The listing builds one solid part. Answer for the finished solid, in the listing's coordinates (mm). A direction names the side the tool comes from. Give positions to 0.01 mm unless a question says otherwise; leave off trailing zeros. Order: outer loops, then holes, each group sorted by start corner. A loop starts at its lowest first (then second) coordinate and runs counter-clockwise, first axis right, second up. Notation, with made-up numbers: (47, 27) - (53, 27) arc R12 cw to (53, 37) - close; hole circle Ø3 at (-23.5, -4.5). An arc over 180 degrees is marked (long way). Use a Markdown table: item, result. Add a question column.
1) Find section A-A, the plane z = 1.25. Determine the outline of the cut face in (x, y), plus the area to 3 significant figures.
2) The mould has two halves that part along Y. Classify faces 1 (the face through (187.854, -58.176, 1.521)), 2 (the face through (50, 98, 3)), 3 (the face through (60, 93, 3)): released by +Y, released by -Y, zero draft, split by the parting line, or undercut.
3) Find section B-B, the plane x = 170.5. Determine the outline of the cut face in (y, z), plus the area to 3 significant figures.
4) Flat-ended cylindrical pins translate along their axes: pin 1 (6 mm diameter, centred on x = 93.5, y = -63.5, fed in from +Z); pin 2 (6 mm diameter, centred on x = 153.5, y = 17, fed in from +Z); pin 3 (3 mm diameter, centred on x = 39.5, y = 57.5, fed in from +Z); pin 4 (0.9 mm diameter, centred on x = 12.5, y = 111, fed in from -Z). Find the tip coordinate at first contact, or state that the pin passes through.
5) Straight lines are drawn through the part: line 1 (Y direction, x = 15.5, z = 6.75); line 2 (Y direction, x = 190, z = 2.2); line 3 (X direction, y = -15.5, z = 4.75). For each, find the intervals that lie inside material, in ascending order.
6) For faces 4 (the face through (122.854, -58.176, 1.521)), 5 (the face through (161, -50, 3)), 6 (the face through (44, 110, 6)), 7 (the face through (47.15, 109.99, 3.71)), 8 (the face through (43.275, 109.449, 5.507)), determine the directions among +Z, -Z, +X, -X, +Y, -Y from which every point of the face is accessible in a straight line to the end or side of a thin tool.
Solid Edge part; units mm, degrees
sketch "Sketch1" plane through (0, 0, 0) normal (0, 0, 1) x (1, 0, 0)
  line L0 (-225, -85) -> (225, -85)
  line L1 (225, -85) -> (225, 85)
  line L2 (225, 85) -> (-225, 85)
  line L3 (-225, 85) -> (-225, -85)
  dimension "D1" = 225
  dimension "D2" = 225
extrude "Protrusion1" add sketch "Sketch1" along normal blind 3
sketch "Sketch2" plane through (0, 0, 3) normal (0, 0, 1) x (1, 0, 0)
  circle A0 centre (-190, 57.5) radius 3
  circle A1 centre (-190, -57.5) radius 3
  circle A2 centre (190, -57.5) radius 3
  circle A3 centre (190, 57.5) radius 3
  dimension "D1" = 190
  dimension "D2" = 190
extrude "Cutout1" cut sketch "Sketch2" against normal through all
sketch "Sketch3" plane through (0, 0, 3) normal (0, 0, 1) x (1, 0, 0)
  circle A0 centre (-15.5, 15.5) radius 2
  circle A1 centre (15.5, 15.5) radius 2
  circle A2 centre (15.5, -15.5) radius 2
  circle A3 centre (-15.5, -15.5) radius 2
  dimension "D1" = 15.5
extrude "Cutout2" cut sketch "Sketch3" against normal through all
sketch "Sketch4" plane through (-112.5, 0, 3) normal (0, 0, 1) x (1, 0, 0)
  circle A0 centre (-12.5, -57.5) radius 3
  dimension "D1" = 12.5
extrude "Cutout3" cut sketch "Sketch4" against normal through all
sketch "Sketch5" plane through (-112.5, 0, 3) normal (0, 0, 1) x (1, 0, 0)
  line L0 (112.5, 85) -> (-52.5, 85)
  line L1 (-52.5, 85) -> (-52.5, -35)
  line L2 (-52.5, -35) -> (112.5, -35)
  line L3 (112.5, -35) -> (112.5, 85)
  dimension "D1" = 52.5
  dimension "D2" = 52.5
extrude "Protrusion2" add sketch "Sketch5" along normal blind 3
sketch "Sketch6" plane through (-112.5, 0, 3) normal (0, 0, 1) x (1, 0, 0)
  circle A0 centre (72.5, -57.5) radius 3
  circle A1 centre (72.5, 57.5) radius 3
extrude "Cutout4" cut sketch "Sketch6" against normal through all
sketch "Sketch7" plane through (-112.5, 0, 0) normal (0, 0, -1) x (1, 0, 0)
  circle A0 centre (97, 15.5) radius 2
  circle A1 centre (97, -15.5) radius 2
  circle A2 centre (72.5, -57.5) radius 3
extrude "Cutout5" cut sketch "Sketch7" against normal through all
mirror "Mirror1" about plane through (0, 0, 0) normal (1, 0, 0) of "Protrusion2", "Cutout3"
mirror "Mirror2" about plane through (0, 0, 0) normal (1, 0, 0) of "Protrusion2", "Cutout3", "Cutout1"
mirror "Mirror3" about plane through (0, 0, 0) normal (1, 0, 0) of "Cutout5", "Cutout4"
sketch "Sketch8" plane through (0, 25, 6) normal (0, 0, 1) x (1, 0, 0)
  line L0 (0, 60) -> (0, -110)
extrude "Cutout8" cut sketch "Sketch8" against normal through all material side at (-0.05, 0, 6)
sketch "Sketch9" plane through (112.5, 0, 0) normal (0, 0, -1) x (1, 0, 0)
  circle A0 centre (-112.5, 0) radius 11
extrude "Cutout9" cut sketch "Sketch9" against normal through all
sketch "Sketch10" plane through (112.5, 0, 3) normal (0, 0, 1) x (-1, 0, 0)
  line L0 (-112.5, 85) -> (112.5, 85)
  line L1 (112.5, 85) -> (112.5, 84)
  line L2 (112.5, 84) -> (-112.5, 84)
  line L3 (-112.5, 84) -> (-112.5, 85)
  dimension "D1" = 112.5
extrude "Cutout10" cut sketch "Sketch10" against normal through all
sketch "Sketch11" plane through (112.5, 85, 3) normal (0, 1, 0) x (-1, 0, 0)
  line L0 (-112.5, -3) -> (112.5, -3)
  line L1 (112.5, -3) -> (112.5, 3)
  line L2 (112.5, 3) -> (-52.5, 3)
  line L3 (-52.5, 3) -> (-52.5, 0)
  line L4 (-52.5, 0) -> (-112.5, 0)
  line L5 (-112.5, 0) -> (-112.5, -3)
extrude "Extrusionsausprägung_4" add sketch "Sketch11" along normal blind 35
sketch "Sketch12" plane through (82.5, 42.5, 6) normal (0, 0, 1) x (0, 1, 0)
  line L0 (77.5, 82.5) -> (-17.7628, -82.5)
  line L1 (-17.7628, -82.5) -> (-3.329, -82.5)
  line L2 (77.5, 57.5) -> (-3.329, -82.5)
  line L3 (77.5, 57.5) -> (77.5, 82.5)
extrude "Extrusionsausschnitt_12" cut sketch "Sketch12" against normal blind 1
sketch "Sketch13" plane through (112.5, 18, 0) normal (0, 0, -1) x (-1, 0, 0)
  line L0 (-112.5, 102) -> (112.5, 102)
  line L1 (112.5, 102) -> (112.5, 92)
  line L2 (112.5, 92) -> (-112.5, 92)
  line L3 (-112.5, 92) -> (-112.5, 102)
  dimension "D1" = 112.5
extrude "Extrusionsausschnitt_13" cut sketch "Sketch13" against normal blind 3
sketch "Sketch14" plane through (82.5, 42.5, 6) normal (0, 0, 1) x (-1, 0, 0)
  circle A0 centre (42.5, -15) radius 3
  circle A1 centre (42.5, -15) radius 2.25
extrude "Protrusion4" add sketch "Sketch14" against normal up to vertex (6 mm away)
sketch "Sketch15" plane through (112.5, 13, 3) normal (0, 0, 1) x (-1, 0, 0)
  circle A0 centre (-77.5, 70.5) radius 2.25
  circle A1 centre (-12.5, 70.5) radius 2.25
  circle A2 centre (72.5, 70.5) radius 2.25
  circle A3 centre (-77.5, -44.5) radius 2.25
  circle A4 centre (-77.5, 70.5) radius 3.4682
  circle A5 centre (-12.5, 70.5) radius 4.4128
  circle A6 centre (72.5, 70.5) radius 5.5704
  circle A7 centre (-77.5, -44.5) radius 3
extrude "Protrusion5" add sketch "Sketch15" against normal up to vertex (3 mm away)
sketch "Sketch16" plane through (82.5, 42.5, 6) normal (0, 0, 1) x (-1, 0, 0)
  circle A0 centre (67, 58) radius 2
  circle A1 centre (67, 58) radius 4
  circle A2 centre (67, 27) radius 4
  circle A3 centre (67, 27) radius 2
extrude "Extrusionsausprägung_7" add sketch "Sketch16" along normal blind 1
sketch "Sketch17" plane through (95, 79.5855, 6) normal (0, 0, 1) x (-1, 0, 0)
  line L0 (-70, -40.4145) -> (95, -40.4145)
  line L1 (95, -40.4145) -> (95, -33.4145)
  line L2 (95, -33.4145) -> (-70, -33.4145)
  line L3 (-70, -33.4145) -> (-70, -40.4145)
  dimension "D1" = 95
extrude "Cutout11" cut sketch "Sketch17" against normal up to next
sketch "Sketch18" plane through (82.5, 39, 6) normal (0, 0, 1) x (-1, 0, 0)
  line L0 (12.5, -74) -> (32.5, -74)
  line L1 (32.5, -74) -> (32.5, -54)
  line L2 (32.5, -54) -> (12.5, -54)
  line L3 (12.5, -54) -> (12.5, -74)
  dimension "D1" = 12.5
  dimension "D2" = 32.5
extrude "Cutout12" cut sketch "Sketch18" against normal through all
fillet "Verrundung_1" radius 10 2 edges at (70, 113, 4.5) (50, 113, 4.5)
properties material "Nylon, allgemein"
The answers:
| question | item | result |
|---|---|---|
| 1 | outline | (0, -84) - (225, -84) - (225, 110) - (72.86, 110) arc R10 ccw to (70, 103) - (70, 93) - (50, 93) - (50, 103) arc R10 ccw to (47.14, 110) - (0, 110) - (0, 11) arc R11 cw to (0, -11) - close; hole circle Ø4 at (15.5, -15.5); hole circle Ø4 at (15.5, 15.5); hole circle Ø4.5 at (40, -57.5); hole circle Ø4.5 at (40, 57.5); hole circle Ø4.5 at (125, -57.5); hole circle Ø4.5 at (190, -57.5); hole circle Ø4.5 at (190, 57.5) |
| 1 | area | 43,000 mm2 |
| 2 | face 1 | undercut |
| 2 | face 2 | zero draft |
| 2 | face 3 | released by +Y |
| 3 | outline | (-84, 0) - (110, 0) - (110, 3) - (-84, 3) - close |
| 3 | area | 582 mm2 |
| 4 | pin 1 | z = 3 |
| 4 | pin 2 | z = 6 |
| 4 | pin 3 | through |
| 4 | pin 4 | z = 3 |
| 5 | line 1 | -19.5 to -17.5, -13.5 to -11.5, 11.5 to 13.5, 17.5 to 19.5 |
| 5 | line 2 | -84 to -59.75, -55.25 to 55.25, 59.75 to 110 |
| 5 | line 3 | 0 to 13.5, 17.5 to 165 |
| 6 | face 4 | +Z, -Z |
| 6 | face 5 | +Z, +X, -Y |
| 6 | face 6 | +Z, +X, -X, +Y, -Y |
| 6 | face 7 | +Z, -Z, +Y |
| 6 | face 8 | +Z |
